Work out the finished part from the listing and answer in its coordinate system (mm). Round coordinates to 2 decimals unless told otherwise and drop trailing zeros. Loops run counter-clockwise (first coordinate to the right, second up) from the corner with the lowest first, then second, coordinate; pieces in that order, holes last. Notation, with made-up numbers: (-5.5, -9) - (-1.5, -9) arc R19 cw to (-1.5, 20) - close; hole circle Ø8 at (54, -9). An arc over 180 degrees is marked (long way). Answer as CSV lines item,"result". Start each with the question number.
Q1. Section A-A on x = 67 is taken. Write down the section's boundary in (y, z), then the cut area to 3 significant figures.
Q2. Section B-B on z = -4.25 is taken. Write down the section's boundary in (x, y).
Q3. Straight lines are drawn through the part: L1, parallel to Z at x = -65, y = -0.1; L2, parallel to Z at x = 56.5, y = -0.6. For each, find the intervals that lie inside material, in ascending order. Write a range as [from, to].
```python
from build123d import *

# Parameters (mm, degrees)
F1_DEPTH  = 0.75
F2_W      = 0.8
F2_H      = 2
F3_DEPTH  = 0.751
F4_W      = 0.8
F4_H      = 2
F5_DEPTH  = 0.751
F6_W      = 0.8
F6_H      = 2
F7_DEPTH  = 0.751
F8_W      = 0.8
F8_H      = 2
F9_DEPTH  = 0.751
F10_W     = 0.8
F10_H     = 2
F11_DEPTH = 0.751
F12_W     = 0.8
F12_H     = 2
F13_DEPTH = 0.751
F14_W     = 0.8
F14_H     = 2
F15_DEPTH = 0.751
F16_W     = 0.8
F16_H     = 2
F17_DEPTH = 0.751
F18_W     = 0.8
F18_H     = 2
F19_DEPTH = 0.751


with BuildPart() as f1:
    # F0 (on Front) → F1 (new body)
    with BuildSketch(Plane.XZ):
        Polygon((89.981408, 0), (-85.018592, 0), (-85.018592, -3), (-55.018592, -3), (-25.518592, -7), (30.481408, -7), (59.981408, -3), (89.981408, -3), align=None)
    extrude(amount=F1_DEPTH)

    # F2 (on face) → F3 (cut, through all)
    with BuildSketch(Plane.XZ.offset(0.75)):
        with Locations((-54.638592, -1)):
            Rectangle(F2_W, F2_H)
    extrude(amount=-F3_DEPTH, mode=Mode.SUBTRACT)

    # F4 (on face) → F5 (cut, through all)
    with BuildSketch(Plane.XZ.offset(0.75)):
        with Locations((-40.638592, -1)):
            Rectangle(F4_W, F4_H)
    extrude(amount=-F5_DEPTH, mode=Mode.SUBTRACT)

    # F6 (on face) → F7 (cut, through all)
    with BuildSketch(Plane.XZ.offset(0.75)):
        with Locations((-25.138592, -1)):
            Rectangle(F6_W, F6_H)
    extrude(amount=-F7_DEPTH, mode=Mode.SUBTRACT)

    # F8 (on face) → F9 (cut, through all)
    with BuildSketch(Plane.XZ.offset(0.75)):
        with Locations((-11.138592, -1)):
            Rectangle(F8_W, F8_H)
    extrude(amount=-F9_DEPTH, mode=Mode.SUBTRACT)

    # F10 (on face) → F11 (cut, through all)
    with BuildSketch(Plane.XZ.offset(0.75)):
        with Locations((2.501408, -1)):
            Rectangle(F10_W, F10_H)
    extrude(amount=-F11_DEPTH, mode=Mode.SUBTRACT)

    # F12 (on face) → F13 (cut, through all)
    with BuildSketch(Plane.XZ.offset(0.75)):
        with Locations((16.101408, -1)):
            Rectangle(F12_W, F12_H)
    extrude(amount=-F13_DEPTH, mode=Mode.SUBTRACT)

    # F14 (on face) → F15 (cut, through all)
    with BuildSketch(Plane.XZ.offset(0.75)):
        with Locations((30.101408, -1)):
            Rectangle(F14_W, F14_H)
    extrude(amount=-F15_DEPTH, mode=Mode.SUBTRACT)

    # F16 (on face) → F17 (cut, through all)
    with BuildSketch(Plane.XZ.offset(0.75)):
        with Locations((44.101408, -1)):
            Rectangle(F16_W, F16_H)
    extrude(amount=-F17_DEPTH, mode=Mode.SUBTRACT)

    # F18 (on face) → F19 (cut, through all)
    with BuildSketch(Plane.XZ.offset(0.75)):
        with Locations((59.601408, -1)):
            Rectangle(F18_W, F18_H)
    extrude(amount=-F19_DEPTH, mode=Mode.SUBTRACT)


solid = f1.part
```
Findings:
1,outline,"(-0.75, -3) - (0, -3) - (0, 0) - (-0.75, 0) - close"
1,area,"2.25 mm^2"
2,outline,"(-45.8, -0.75) - (50.76, -0.75) - (50.76, 0) - (-45.8, 0) - close"
3,L1,"z = [-3, 0]"
3,L2,"z = [-3.47, 0]"
